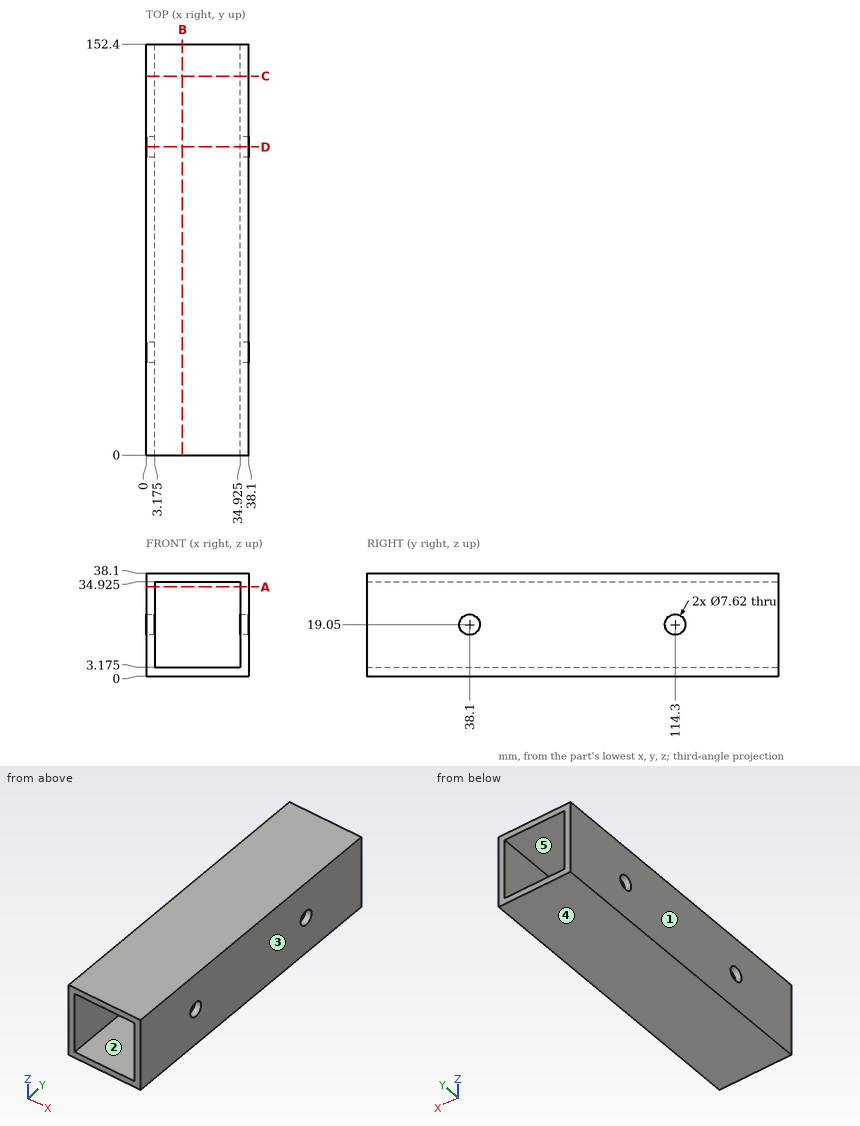
Answer from the drawing. Dimensions are ordinates in mm from the lowest x, y and z of the part. A direction names the side the tool comes from. Give positions to 0.01 mm unless a question says otherwise; leave off trailing zeros. Loops run counter-clockwise (first coordinate to the right, second up) from the corner with the lowest first, then second, coordinate; pieces in that order, holes last. Notation, with made-up numbers: (37, 75.5) - (67, 75.5) arc R22 ccw to (67, 86.5) - close; hole circle Ø8 at (-21, -40). An arc over 180 degrees is marked (long way). Answer as CSV lines item,"result". Start each with the question number.
Item 1: A cutting plane is placed at A-A on z = 33. Determine the outline of the cut face in (x, y) (3 decimals), then the cut area to 3 significant figures.
Item 2: For the marked faces 1 and 2, determine the directions among +Z, -Z, +X, -X, +Y, -Y from which every point of the face is accessible in a straight line to the end or side of a thin tool.
Item 3: A cutting plane is placed at C-C on y = 140.5. Determine the outline of the cut face in (x, z) (3 decimals), then the cut area to 3 significant figures.
Item 4: A cutting plane is placed at B-B on x = 13.5. Determine the outline of the cut face in (y, z) (3 decimals), then the cut area to 3 significant figures.
Item 5: This flat-tipped pin is pushed along its axis until it touches: pin 1 (6 mm diameter, centred on x = 29, z = 23.5, fed in from -Y). Where does it stop, or does it pass through?
Item 6: The mould has two halves that part along X. Classify the marked faces 3, 4 and 5: +X half, -X half, draft (parallel to the pull), parting line (faces both ways), or undercut.
Item 7: A cutting plane is placed at D-D on y = 114.3. Determine the outline of the cut face in (x, z) (3 decimals), then the cut area to 3 significant figures.
Item 8: Find the intervals of material crossed by line 1 (Y direction, x = 37, z = 19.05); line 2 (X direction, y = 60, z = 17) (3 decimals); line 3 (Z direction, x = 2, y = 114), in increasing order. Write a range as from..to.
Found:
1,outline,"(0, 0) - (3.175, 0) - (3.175, 152.4) - (0, 152.4) - close; (34.925, 0) - (38.1, 0) - (38.1, 152.4) - (34.925, 152.4) - close"
1,area,"968 mm^2"
2,face 1,"+Z, -Z, -X, +Y, -Y"
2,face 2,"+Y, -Y"
3,outline,"(0, 0) - (38.1, 0) - (38.1, 38.1) - (0, 38.1) - close; hole (3.175, 3.175) - (34.925, 3.175) - (34.925, 34.925) - (3.175, 34.925) - close"
3,area,"444 mm^2"
4,outline,"(0, 0) - (152.4, 0) - (152.4, 3.175) - (0, 3.175) - close; (0, 34.925) - (152.4, 34.925) - (152.4, 38.1) - (0, 38.1) - close"
4,area,"968 mm^2"
5,pin 1,"passes through"
6,face 3,"+X half"
6,face 4,"draft"
6,face 5,"undercut"
7,outline,"(0, 0) - (38.1, 0) - (38.1, 15.24) - (34.925, 15.24) - (34.925, 3.175) - (3.175, 3.175) - (3.175, 15.24) - (0, 15.24) - close; (0, 22.86) - (3.175, 22.86) - (3.175, 34.925) - (34.925, 34.925) - (34.925, 22.86) - (38.1, 22.86) - (38.1, 38.1) - (0, 38.1) - close"
7,area,"395 mm^2"
8,line 1,"y = 0..34.29, 41.91..110.49, 118.11..152.4"
8,line 2,"x = 0..3.175, 34.925..38.1"
8,line 3,"z = 0..15.25, 22.85..38.1"
